For this review, take the finished solid that the model builds, in its own axes (mm). Coordinates: 2 decimals unless noted, no trailing zeros. Loops run counter-clockwise (first coordinate to the right, second up) from the corner with the lowest first, then second, coordinate; pieces in that order, holes last. Notation, with made-up numbers: (-3.5, 2.5) -> (33.5, 2.5) arc R19 ccw to (33.5, 22.5) -> close; hole circle Ø4 at (40, 53). An arc over 180 degrees is marked (long way). Use a Markdown table: item, result.
from build123d import *

# Parameters (mm, degrees)
ESQUISSE1_R        = 12.5
ESQUISSE1_R_2      = 10
BOSS_EXTRU_1_DEPTH = 5
CONG_1_R           = 0.5


with BuildPart() as part:
    # Esquisse1 → Boss.-Extru.1 (new body)
    with BuildSketch(Plane(origin=(0, 0, 0), x_dir=(1, 0, 0), z_dir=(0, 1, 0))):
        with Locations(Location((0, 0, 0), (0, 0, 270))):
            Circle(ESQUISSE1_R)
        with Locations(Location((0, 0, 0), (0, 0, 270))):
            Circle(ESQUISSE1_R_2, mode=Mode.SUBTRACT)
    extrude(amount=BOSS_EXTRU_1_DEPTH)

    # Congé1
    cong_1_edges = [part.edges().sort_by_distance(p)[0] for p in [
        (0, 0, -12.5),
        (0, 5, -12.5),
        (0, 0, -10),
        (0, 5, -10),
    ]]
    fillet(cong_1_edges, radius=CONG_1_R)


solid = part.part
(1) Take a section at B-B on x = 0. Write out the cut boundary in (y, z).
Found:
| item | result |
|---|---|
| outline | (0, -12) arc R0.5 ccw to (0.5, -12.5) -> (4.5, -12.5) arc R0.5 ccw to (5, -12) -> (5, -10.5) arc R0.5 ccw to (4.5, -10) -> (0.5, -10) arc R0.5 ccw to (0, -10.5) -> close; (0, 10.5) arc R0.5 ccw to (0.5, 10) -> (4.5, 10) arc R0.5 ccw to (5, 10.5) -> (5, 12) arc R0.5 ccw to (4.5, 12.5) -> (0.5, 12.5) arc R0.5 ccw to (0, 12) -> close |
(2) Take a section at C-C on y = 4.05. Write out the cut boundary in (x, z), plus the area to 3 significant figures.
Found:
| item | result |
|---|---|
| outline | circle Ø25 at (0, 0); hole circle Ø20 at (0, 0) |
| area | 177 mm^2 |
(3) Take a section at A-A on z = 0. Write out the cut boundary in (x, y), plus the area to 3 significant figures.
Found:
| item | result |
|---|---|
| outline | (-12.5, 0.5) arc R0.5 ccw to (-12, 0) -> (-10.5, 0) arc R0.5 ccw to (-10, 0.5) -> (-10, 4.5) arc R0.5 ccw to (-10.5, 5) -> (-12, 5) arc R0.5 ccw to (-12.5, 4.5) -> close; (10, 0.5) arc R0.5 ccw to (10.5, 0) -> (12, 0) arc R0.5 ccw to (12.5, 0.5) -> (12.5, 4.5) arc R0.5 ccw to (12, 5) -> (10.5, 5) arc R0.5 ccw to (10, 4.5) -> close |
| area | 24.6 mm^2 |
(4) Mouldability with a two-part tool opening along X and no side actions: class faces 1 (the face through (-9.76, 2.47, -2.17)), 2 (the face through (-11, 0, 0)), 3 (the face through (3.755, 2.472, 11.923)) as pulls with the +X half, pulls with the -X half, needs draft (parallel to the pull), parting line crosses it, or undercut.
Found:
| item | result |
|---|---|
| face 1 | undercut |
| face 2 | needs draft |
| face 3 | parting line crosses it |
(5) For line 1 along X through (y, z) = (3.45, 0); line 2 along Z through (x, y) = (-0.5, 4.7); line 3 along Y through (x, z) = (-9, -8), list the stretches that pass through material, from the lowest coordinate up.
Found:
| item | result |
|---|---|
| line 1 | x = -12.5 to -10, 10 to 12.5 |
| line 2 | z = -12.45 to -10.03, 10.03 to 12.45 |
| line 3 | y = 0 to 5 |
(6) For pin 1 Ø2 at (x, y) = (1.5, 2.5) entering from +Z, flat-tipped, find the tip position at first contact; note if it passes through.
Found:
| item | result |
|---|---|
| pin 1 | stops at z = 12.49 |
